CAD build for the part. Positions are in the model's coordinates, mm. Coordinates: 2 decimals unless noted, no trailing zeros. Write each loop counter-clockwise with the first axis right and the second up, starting at its lowest first coordinate (ties: lowest second). Pieces come first, ordered by that corner, then holes.
```python
from build123d import *

# Parameters (mm, degrees)
SKETCH2_W                = 100
SKETCH2_H                = 100
BOSS_EXTRUDE1_DEPTH      = 1.5875
CUT_EXTRUDE1_DEPTH       = 5
SKETCH4_R                = 1.25
CUT_EXTRUDE2_DEPTH       = 5
CUT_EXTRUDE4_DEPTH       = 5
CUT_EXTRUDE6_DEPTH       = 5
CIRPATTERN1_COUNT        = 4
CIRPATTERN4_COUNT        = 4
FILLET2_R                = 2
F_2_5MM_DOWEL_HOLE1_D    = 2.5
F_2_5MM_DOWEL_HOLE2_D    = 2.5
F_9_0_9_DIAMETER_HOLE1_D = 9
CIRPATTERN5_COUNT        = 4


with BuildPart() as part:
    # Sketch2 → Boss-Extrude1 (new body)
    with BuildSketch(Plane(origin=(0, 0, 0), x_dir=(1, 0, 0), z_dir=(0, 1, 0))):
        with Locations((50, 50)):
            Rectangle(SKETCH2_W, SKETCH2_H)
    extrude(amount=BOSS_EXTRUDE1_DEPTH)

    # Sketch3 → Cut-Extrude1 (cut)
    with BuildSketch(Plane(origin=(0, 1.5875, 0), x_dir=(1, 0, 0), z_dir=(0, 1, 0))):
        with BuildLine():
            Line((11.25, 80), (11.25, 20))
            ThreePointArc((11.25, 20), (10, 18.75), (8.75, 20))
            Line((8.75, 20), (8.75, 80))
            ThreePointArc((8.75, 80), (10, 81.25), (11.25, 80))
        make_face()
    cut_extrude1 = extrude(amount=-CUT_EXTRUDE1_DEPTH, mode=Mode.SUBTRACT)

    # Sketch4 → Cut-Extrude2 (cut)
    with BuildSketch(Plane(origin=(0, 1.5875, 0), x_dir=(1, 0, 0), z_dir=(0, 1, 0))):
        with Locations((10, 10)):
            Circle(SKETCH4_R)
    cut_extrude2 = extrude(amount=-CUT_EXTRUDE2_DEPTH, mode=Mode.SUBTRACT)

    # Sketch6 → Cut-Extrude4 (cut)
    with BuildSketch(Plane(origin=(0, 1.5875, 0), x_dir=(1, 0, 0), z_dir=(0, 1, 0))):
        with BuildLine():
            Line((49.25, 11.25), (50.75, 11.25))
            ThreePointArc((50.75, 11.25), (52, 10), (50.75, 8.75))
            Line((50.75, 8.75), (49.25, 8.75))
            ThreePointArc((49.25, 8.75), (48, 10), (49.25, 11.25))
        make_face()
    cut_extrude4 = extrude(amount=-CUT_EXTRUDE4_DEPTH, mode=Mode.SUBTRACT)

    # Sketch8 → Cut-Extrude6 (cut)
    with BuildSketch(Plane(origin=(0, 1.5875, 0), x_dir=(1, 0, 0), z_dir=(0, 1, 0))):
        with BuildLine():
            Line((30, 51.25), (40, 51.25))
            ThreePointArc((40, 51.25), (41.25, 50), (40, 48.75))
            Line((40, 48.75), (30, 48.75))
            ThreePointArc((30, 48.75), (28.75, 50), (30, 51.25))
        make_face()
    cut_extrude6 = extrude(amount=-CUT_EXTRUDE6_DEPTH, mode=Mode.SUBTRACT)

    # Mirror3: Cut-Extrude1 across plane
    add(cut_extrude1.mirror(Plane(origin=(50, 0, 0), x_dir=(0, 0, 1), z_dir=(1, 0, 0))), mode=Mode.SUBTRACT)

    # CirPattern1: Cut-Extrude6 ×4 about axis
    cirpattern1_axis = Axis((50, 0, -50), (0, 1, 0))
    for i in range(1, CIRPATTERN1_COUNT):
        add(cut_extrude6.rotate(cirpattern1_axis, i * 360 / CIRPATTERN1_COUNT), mode=Mode.SUBTRACT)

    # CirPattern4: Cut-Extrude2 ×4 about axis
    cirpattern4_axis = Axis((50, 0, -50), (0, 1, 0))
    for i in range(1, CIRPATTERN4_COUNT):
        add(cut_extrude2.rotate(cirpattern4_axis, i * 360 / CIRPATTERN4_COUNT), mode=Mode.SUBTRACT)

    # Mirror6: Cut-Extrude4 across plane
    add(cut_extrude4.mirror(Plane(origin=(0, 0, -50), x_dir=(1, 0, 0), z_dir=(0, 0, -1))), mode=Mode.SUBTRACT)

    # Fillet2
    fillet2_edges = [part.edges().sort_by_distance(p)[0] for p in [
        (0, 0.79375, 0),
        (100, 0.79375, 0),
        (100, 0.79375, -100),
        (0, 0.79375, -100),
    ]]
    fillet(fillet2_edges, radius=FILLET2_R)

    # 2.5mm Dowel Hole1 (through all)
    with Locations(Plane(origin=(0, 1.5875, 0), x_dir=(1, 0, 0), z_dir=(0, 1, 0))):
        with Locations((62.5, 15), (37.5, 15)):
            Hole(F_2_5MM_DOWEL_HOLE1_D / 2)

    # 2.5mm Dowel Hole2 (through all)
    with Locations(Plane(origin=(0, 1.5875, 0), x_dir=(1, 0, 0), z_dir=(0, 1, 0))):
        with Locations((42.7, 59.4), (67.7, 59.4)):
            Hole(F_2_5MM_DOWEL_HOLE2_D / 2)

    # 9.0 _9_ Diameter Hole1 (through all)
    with Locations(Plane(origin=(0, 1.5875, 0), x_dir=(1, 0, 0), z_dir=(0, 1, 0))):
        with Locations((80, 20)):
            f_9_0_9_diameter_hole1 = Hole(F_9_0_9_DIAMETER_HOLE1_D / 2)

    # CirPattern5: 9.0 _9_ Diameter Hole1 ×4 about axis
    cirpattern5_axis = Axis((50, 0, -50), (0, 1, 0))
    for i in range(1, CIRPATTERN5_COUNT):
        add(f_9_0_9_diameter_hole1.rotate(cirpattern5_axis, i * 360 / CIRPATTERN5_COUNT), mode=Mode.SUBTRACT)


solid = part.part
```
Item 1: Flat gauge pin, fed straight in: pin 1 Ø3 at (x, z) = (10, -10) entering from -Y. Where does the tip first touch, or does it go through?
Item 2: Saw through at D-D, the plane x = 67.7. Write the cut outline in (y, z).
Item 3: Saw through at A-A, the plane z = -50. Write the cut outline in (x, y), and give its area (3 significant figures).
Item 4: Wall check: line 1 along X through (y, z) = (1, -64); line 2 along X through (y, z) = (0.4, -90); line 3 along Z through (x, y) = (31, 0.8). Give the ranges that are in metal, low to high.
Item 5: Saw through at C-C, the plane z = -64.5. Write the cut outline in (x, y), and give its area (3 significant figures).
Item 6: Two-plate mould, pull along Z, no slides. Class faces 1 (the flat face through (49, 0, -51)), 2 (the cylindrical face through (84.496, 0.783, -20.198)): +Z half, -Z half, draft (parallel to the pull), parting line (faces both ways), or undercut.
Item 7: Saw through at B-B, the plane x = 10. Write the cut outline in (y, z), and give its area (3 significant figures).
Working result:
1. pin 1: stops at y = 0
2. outline: (0, -100) - (1.59, -100) - (1.59, -60.65) - (0, -60.65) - close; (0, -58.15) - (1.59, -58.15) - (1.59, -51.25) - (0, -51.25) - close; (0, -48.75) - (1.59, -48.75) - (1.59, 0) - (0, 0) - close
3. outline: (0, 0) - (8.75, 0) - (8.75, 1.59) - (0, 1.59) - close; (11.25, 0) - (28.75, 0) - (28.75, 1.59) - (11.25, 1.59) - close; (41.25, 0) - (58.75, 0) - (58.75, 1.59) - (41.25, 1.59) - close; (71.25, 0) - (88.75, 0) - (88.75, 1.59) - (71.25, 1.59) - close; (91.25, 0) - (100, 0) - (100, 1.59) - (91.25, 1.59) - close
3. area: 111 mm2
4. line 1: x = 0 to 8.75, 11.25 to 48.75, 51.25 to 88.75, 91.25 to 100
4. line 2: x = 0 to 8.75, 11.25 to 48, 52 to 88.75, 91.25 to 100
4. line 3: z = -100 to -51.25, -48.75 to 0
5. outline: (0, 0) - (8.75, 0) - (8.75, 1.59) - (0, 1.59) - close; (11.25, 0) - (48.75, 0) - (48.75, 1.59) - (11.25, 1.59) - close; (51.25, 0) - (88.75, 0) - (88.75, 1.59) - (51.25, 1.59) - close; (91.25, 0) - (100, 0) - (100, 1.59) - (91.25, 1.59) - close
5. area: 147 mm2
6. face 1: draft
6. face 2: undercut
7. outline: (0, -100) - (1.59, -100) - (1.59, -91.25) - (0, -91.25) - close; (0, -88.75) - (1.59, -88.75) - (1.59, -81.25) - (0, -81.25) - close; (0, -18.75) - (1.59, -18.75) - (1.59, -11.25) - (0, -11.25) - close; (0, -8.75) - (1.59, -8.75) - (1.59, 0) - (0, 0) - close
7. area: 51.6 mm2
